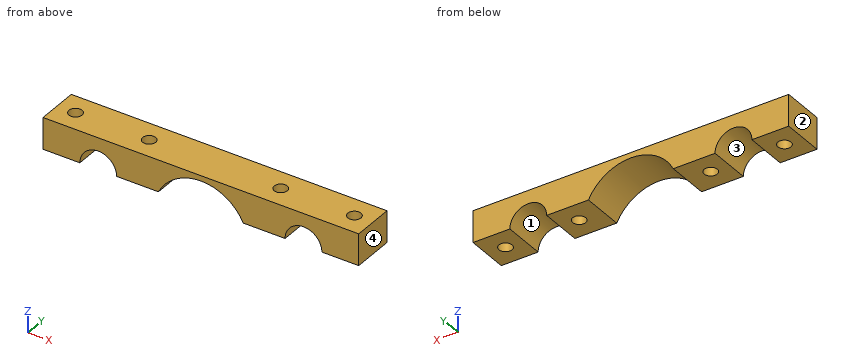
```python
from build123d import *

# Parameters (mm, degrees)
F1_DEPTH = 8
F3_D     = 5


with BuildPart() as f1:
    # F0 (on Front) → F1 (new body, symmetric)
    with BuildSketch(Plane.XZ):
        with BuildLine():
            Line((-60, -6), (-46, -6))
            ThreePointArc((-46, -6), (-39, 1), (-32, -6))
            Line((-32, -6), (-16.124515, -6))
            ThreePointArc((-16.124515, -6), (0, 4), (16.124515, -6))
            Line((16.124515, -6), (32, -6))
            ThreePointArc((32, -6), (39, 1), (46, -6))
            Line((46, -6), (60, -6))
            Line((60, -6), (60, 6))
            Line((60, 6), (-60, 6))
            Line((-60, 6), (-60, -6))
        make_face()
    extrude(amount=F1_DEPTH, both=True)

    # F3 (through all)
    with Locations(Plane.XY.offset(6)):
        with Locations((-53, 0), (-25, 0), (25, 0), (53, 0)):
            Hole(F3_D / 2)


solid = f1.part
```
Verification items for the finished model (mm, model axes). Face numbers are marked on the shaded views. Coordinates: 2 decimals unless noted, no trailing zeros. Write each loop counter-clockwise with the first axis right and the second up, starting at its lowest first coordinate (ties: lowest second). Pieces come first, ordered by that corner, then holes. Notation, with made-up numbers: M 66,68.5 L 85,68.5 A17 cw 85,72.5 Z; hole C 58.25,85 d7. An arc over 180 degrees is marked long. Answer as a JSON object with one key per item and string values. Group by question number.
(1) Release check for a two-part mould opening along X. For the marked faces 1, 2, 3 and 4 record: +X half, -X half, draft (parallel to the pull), parting line (faces both ways), or undercut.
(2) Cross-section at C-C, the plane x = 53. Record the cut outline in (y, z).
(3) Gauge pin test, flat end, axial feed: pin 1 (6 mm diameter, centred on x = -25, y = 0, fed in from -Z). Record the tip position at first contact, or that the pin passes through.
(4) Cross-section at B-B, the plane y = 0. Record the cut outline in (x, z), and give its area (3 significant figures).
(5) Cross-section at D-D, the plane x = -23.5. Record the cut outline in (y, z), and give its area (3 significant figures).
(6) Material ranges on line 1 (Y direction, x = 53, z = -2); line 2 (X direction, y = 4.5, z = -3.5); line 3 (X direction, y = -6.25, z = -4.5), recorded low to high.
(7) Cross-section at A-A, the plane z = -1.75. Record the cut outline in (x, y).
Reply:
{
 "1": {"face 1": "undercut", "face 2": "-X half", "face 3": "undercut", "face 4": "+X half"},
 "2": {"outline": "M -8,-6 L -2.5,-6 L -2.5,6 L -8,6 Z; M 2.5,-6 L 8,-6 L 8,6 L 2.5,6 Z"},
 "3": {"pin 1": "z = -6"},
 "4": {"outline": "M -60,-6 L -55.5,-6 L -55.5,6 L -60,6 Z; M -50.5,-6 L -46,-6 A7 cw -32,-6 L -27.5,-6 L -27.5,6 L -50.5,6 Z; M -22.5,-6 L -16.12,-6 A18 cw 16.12,-6 L 22.5,-6 L 22.5,6 L -22.5,6 Z; M 27.5,-6 L 32,-6 A7 cw 46,-6 L 50.5,-6 L 50.5,6 L 27.5,6 Z; M 55.5,-6 L 60,-6 L 60,6 L 55.5,6 Z", "area": "815 mm²"},
 "5": {"outline": "M -8,-6 L -2,-6 L -2,6 L -8,6 Z; M 2,-6 L 8,-6 L 8,6 L 2,6 Z", "area": "144 mm²"},
 "6": {"line 1": "-8 to -2.5, 2.5 to 8", "line 2": "-60 to -45.54, -32.46 to -14.62, 14.62 to 32.46, 45.54 to 60", "line 3": "-60 to -45.84, -32.16 to -15.29, 15.29 to 32.16, 45.84 to 60"},
 "7": {"outline": "M -60,-8 L -44.56,-8 L -44.56,8 L -60,8 Z; M -33.44,-8 L -13.19,-8 L -13.19,8 L -33.44,8 Z; M 13.19,-8 L 33.44,-8 L 33.44,8 L 13.19,8 Z; M 44.56,-8 L 60,-8 L 60,8 L 44.56,8 Z; hole C -53,0 d5; hole C -25,0 d5; hole C 25,0 d5; hole C 53,0 d5"}
}
